```python
from build123d import *

# Parameters (mm, degrees)
SKETCH1_W               = 50
SKETCH1_H               = 16
BOSS_EXTRUDE1_DEPTH     = 2
SKETCH2_R               = 2.325
BOSS_EXTRUDE2_DEPTH     = 8
SKETCH3_W               = 50
SKETCH3_H               = 2
BOSS_EXTRUDE3_DEPTH     = 12
SKETCH4_W               = 4.2
SKETCH4_H               = 50
BOSS_EXTRUDE4_DEPTH     = 20
CUT_EXTRUDE1_DEPTH      = 121.124312029
CUT_EXTRUDE1_DEPTH_BACK = 4.2
SKETCH7_R               = 8
SKETCH8_W               = 16
SKETCH8_H               = 10
CUT_EXTRUDE2_DEPTH      = 4.2
FILLET1_R               = 3
SKETCH9_W               = 3.5
SKETCH9_H               = 10
CUT_EXTRUDE4_DEPTH      = 10


with BuildPart() as part:
    # Sketch1 → Boss-Extrude1 (new body)
    with BuildSketch(Plane(origin=(0, 0, 0), x_dir=(0, 0, -1), z_dir=(1, 0, 0))):
        with Locations((87.541975563, 21.779240865)):
            Rectangle(SKETCH1_W, SKETCH1_H)
    extrude(amount=BOSS_EXTRUDE1_DEPTH)

    # Sketch2 → Boss-Extrude2 (add)
    with BuildSketch(Plane.ZY):
        with Locations((-107.933354654, 21.779240865)):
            Circle(SKETCH2_R)
        with Locations((-67.933354654, 21.779240865)):
            Circle(SKETCH2_R)
    extrude(amount=BOSS_EXTRUDE2_DEPTH)

    # Sketch3 → Boss-Extrude3 (add)
    with BuildSketch(Plane(origin=(2, 0, 0), x_dir=(0, 0, -1), z_dir=(1, 0, 0))):
        with Locations((87.541975563, 14.779240865)):
            Rectangle(SKETCH3_W, SKETCH3_H)
    extrude(amount=BOSS_EXTRUDE3_DEPTH)

    # Sketch4 → Boss-Extrude4 (add)
    with BuildSketch(Plane(origin=(0, 15.779240865, 0), x_dir=(1, 0, 0), z_dir=(0, 1, 0))):
        with Locations((11.9, 87.541975563)):
            Rectangle(SKETCH4_W, SKETCH4_H)
    extrude(amount=BOSS_EXTRUDE4_DEPTH)

    # Sketch7 → Cut-Extrude1 (cut, two sides: drawn at the far end of the back side and taken through both)
    with BuildSketch(Plane(origin=(14, 0, 0), x_dir=(0, 0, -1), z_dir=(1, 0, 0)).offset(-CUT_EXTRUDE1_DEPTH_BACK)):
        with Locations(Location((74.041975563, 25.779240865, 0), (0, 0, 180))):
            Circle(SKETCH7_R)
        with Locations(Location((101.041975563, 25.779240865, 0), (0, 0, 180))):
            Circle(SKETCH7_R)
    extrude(amount=CUT_EXTRUDE1_DEPTH + CUT_EXTRUDE1_DEPTH_BACK, mode=Mode.SUBTRACT)

    # Sketch8 → Cut-Extrude2 (cut)
    with BuildSketch(Plane(origin=(14, 0, 0), x_dir=(0, 0, -1), z_dir=(1, 0, 0))):
        with Locations((74.041975563, 30.779240865)):
            Rectangle(SKETCH8_W, SKETCH8_H)
        with Locations((101.041975563, 30.779240865)):
            Rectangle(SKETCH8_W, SKETCH8_H)
    extrude(amount=-CUT_EXTRUDE2_DEPTH, mode=Mode.SUBTRACT)

    # Fillet1
    fillet1_edges = [part.edges().sort_by_distance(p)[0] for p in [
        (1, 29.779240865, -62.541975563),
        (1, 29.779240865, -112.541975563),
    ]]
    fillet(fillet1_edges, radius=FILLET1_R)

    # Sketch9 → Cut-Extrude4 (cut)
    with BuildSketch(Plane(origin=(14, 0, 0), x_dir=(0, 0, -1), z_dir=(1, 0, 0))):
        with Locations((64.291975563, 30.779240865)):
            Rectangle(SKETCH9_W, SKETCH9_H)
        with Locations((110.791975563, 30.779240865)):
            Rectangle(SKETCH9_W, SKETCH9_H)
    extrude(amount=-CUT_EXTRUDE4_DEPTH, mode=Mode.SUBTRACT)


solid = part.part
```
Geometry check sheet. Reference: the model listing, model coordinates, mm. A direction names the side the tool comes from. Coordinates: 2 decimals unless noted, no trailing zeros. Write each loop counter-clockwise with the first axis right and the second up, starting at its lowest first coordinate (ties: lowest second). Pieces come first, ordered by that corner, then holes. Notation, with made-up numbers: M 80.5,21.25 L 86.5,21.25 A12 cw 86.5,43.25 Z; hole C 41.5,61 d5. An arc over 180 degrees is marked long. One line per item, written item: value. Start each with the question number.
(1) Sectioned sample at C-C, the plane y = 29. Enter the section's corners in (x, z) (3 decimals), and give its area (3 significant figures).
(2) Scan lines: line 1 along X through (y, z) = (23.25, -87); line 2 along X through (y, z) = (22, -77); line 3 along Y through (x, z) = (3, -66). Record each from-to range of solid material in increasing order. Write a range as [from, to].
(3) Sectioned sample at D-D, the plane y = 18.75. Enter the section's corners in (x, z), and give its area (3 significant figures).
(4) Tool access check on faces 5 (the face through (12, 31, -93.042)), 6 (the face through (2, 23, -87)), 7 (the face through (12, 25.779, -64)). Record the directions out of +Z, -Z, +X, -X, +Y, -Y that give a thin tool (end or side, any length) a straight path to the whole face; none if there is none.
(5) Depth check by flat-ended pin: pin 1 (1.5 mm diameter, centred on x = 5.5, z = -89.5, fed in from +Y); pin 2 (1.5 mm diameter, centred on y = 22, z = -104.5, fed in from -X); pin 3 (1 mm diameter, centred on x = 12.5, z = -110, fed in from +Y). Enter the tip coordinate at first touch or a pass-through.
(6) Release check for a two-part mould opening along Z. For faces 1 (the face through (1.01, 28.88, -63.4)), 2 (the face through (14, 22, -87)), 3 (the face through (0, 22, -87)), 4 (the face through (11.87, 17.78, -73.87)) record: released by +Z, released by -Z, zero draft, split by the parting line, or undercut.
(7) Sectioned sample at A-A, the plane z = -91. Enter the section's corners in (x, y).
(8) Sectioned sample at B-B, the plane x = 11. Enter the section's corners in (y, z).
Filled sheet:
1. outline: M 0,-111.559 L 2,-111.559 L 2,-63.525 L 0,-63.525 Z; M 9.8,-93.042 L 14,-93.042 L 14,-82.042 L 9.8,-82.042 Z
1. area: 142 mm²
2. line 1: [0, 2], [9.8, 14]
2. line 2: [0, 2]
2. line 3: [13.78, 15.78]
3. outline: M 0,-112.54 L 2,-112.54 L 2,-62.54 L 0,-62.54 Z; M 9.8,-112.54 L 14,-112.54 L 14,-104.86 L 9.8,-104.86 Z; M 9.8,-97.22 L 14,-97.22 L 14,-77.86 L 9.8,-77.86 Z; M 9.8,-70.22 L 14,-70.22 L 14,-62.54 L 9.8,-62.54 Z
3. area: 246 mm²
4. face 5: -Z, +X, +Y
4. face 6: +Z, -Z, +Y
4. face 7: +Z, +X, +Y
5. pin 1: y = 15.78
5. pin 2: x = 0
5. pin 3: y = 25.78
6. face 1: released by +Z
6. face 2: zero draft
6. face 3: undercut
6. face 4: undercut
7. outline: M 0,13.78 L 14,13.78 L 14,35.78 L 9.8,35.78 L 9.8,15.78 L 2,15.78 L 2,29.78 L 0,29.78 Z
8. outline: M 13.78,-112.54 L 25.78,-112.54 L 25.78,-109.04 A8 cw 25.78,-93.04 L 35.78,-93.04 L 35.78,-82.04 L 25.78,-82.04 A8 cw 25.78,-66.04 L 25.78,-62.54 L 13.78,-62.54 Z
